Could you check a few things on this model? Use its own coordinates, in mm. A direction names the side the tool comes from. Coordinates: 2 decimals unless noted, no trailing zeros. Write each loop counter-clockwise with the first axis right and the second up, starting at its lowest first coordinate (ties: lowest second). Pieces come first, ordered by that corner, then holes. Notation, with made-up numbers: (1.25, 45) - (11.25, 45) arc R12 cw to (11.25, 54) - close; hole circle Ø9 at (78, 6). An arc over 180 degrees is marked (long way). Answer as a JSON object with one key per item and string values. Group by question number.
1) Will these pins go through, and if not, where does the flat tip stop? pin 1 Ø0.8 at (x, z) = (0, -2) entering from -Y; pin 2 Ø2 at (x, z) = (5, 2) entering from -Y; pin 3 Ø2 at (y, z) = (-5.5, -8) entering from +X.
2) We'd pull the mould along Z, two halves only. Please class faces 1 (the cylindrical face through (3.4, -4.1, 4.4)), 2 (the flat face through (0, -3, -10.5)), 3 (the flat face through (0, -7.5, -9)): released by +Z, released by -Z, zero draft, split by the parting line, or undercut.
3) If we section it at B-B (z = 4.5): Write out the boundary of the cut face in (x, y) (3 decimals), plus the area to 3 significant figures.
4) Please list where these lines run through material, in increasing order: line 1 along Z through (x, y) = (0, -5); line 2 along X through (y, z) = (-3.5, 6.25); line 3 along X through (y, z) = (-0.25, -4.75).
5) On a 3-axis mill with a long thin cutter (end or side, diameter ignored), from which of +Z, -Z, +X, -X, +Y, -Y can I reach the whole of each face in a straight line? I mean faces 4 (the flat face through (5, -0.8, 0)), 5 (the flat face through (0, -7.5, 9)), 6 (the flat face through (-5, -0.8, 0)), 7 (the cylindrical face through (1.5, -7.39, -4.44)). Say none if no direction works.
6) If we section it at D-D (y = -3.5): Write out the boundary of the cut face in (x, z).
7) If we section it at C-C (z = -9): Write out the boundary of the cut face in (x, y).
8) If we section it at A-A (x = 0): Write out the boundary of the cut face in (y, z) (3 decimals), plus the area to 3 significant figures.
```python
from build123d import *

# Parameters (mm, degrees)
EXTRUDE_1_DEPTH             = 10.5
FILLET_1_R                  = 0.3
FILLET_2_R                  = 2
HOLE_WIZARD_M82_D           = 6.8
HOLE_WIZARD_M82_CSINK_D     = 8.05
HOLE_WIZARD_M82_CSINK_ANGLE = 90


with BuildPart() as part:
    # Эскиз1 → Бобышка-Вытянуть1 (new body, symmetric)
    with BuildSketch(Plane.XY):
        with BuildLine():
            Line((-4, 0), (4, 0))
            Line((4, 0), (4, -0.8))
            Line((4, -0.8), (6.5, -0.8))
            Line((6.5, -0.8), (6.5, -1.6))
            ThreePointArc((6.5, -1.6), (4.386776199, -4.87777644), (1.5, -7.5))
            Line((1.5, -7.5), (-1.5, -7.5))
            ThreePointArc((-1.5, -7.5), (-4.386776199, -4.87777644), (-6.5, -1.6))
            Line((-6.5, -1.6), (-6.5, -0.8))
            Line((-6.5, -0.8), (-4, -0.8))
            Line((-4, -0.8), (-4, 0))
        make_face()
    extrude(amount=EXTRUDE_1_DEPTH, both=True)

    # Скругление1
    fillet_1_edges = [part.edges().sort_by_distance(p)[0] for p in [
        (6.5, -0.8, 0),
        (6.5, -1.6, 0),
        (-6.5, -1.6, 0),
        (-6.5, -0.8, 0),
        (-4, 0, 0),
        (4, 0, 0),
    ]]
    fillet(fillet_1_edges, radius=FILLET_1_R)

    # Скругление2
    fillet_2_edges = [part.edges().sort_by_distance(p)[0] for p in [
        (1.5, -7.5, 0),
        (-1.5, -7.5, 0),
    ]]
    fillet(fillet_2_edges, radius=FILLET_2_R)

    # Отверстие обработанное метчиком M82 (through all)
    with Locations(Plane(origin=(0, 0, 0), x_dir=(1, 0, 0), z_dir=(0, 1, 0))):
        with Locations((0, -4.5)):
            CounterSinkHole(HOLE_WIZARD_M82_D / 2, HOLE_WIZARD_M82_CSINK_D / 2, counter_sink_angle=HOLE_WIZARD_M82_CSINK_ANGLE)

    # Эскиз5 → Повернуть1 (revolve)
    with BuildSketch(Plane(origin=(0, 0, 0), x_dir=(0, 0, -1), z_dir=(1, 0, 0))):
        with BuildLine():
            Line((6.5, -4.3), (6.5, -8.3))
            ThreePointArc((6.5, -8.3), (4.5, -6.3), (6.5, -4.3))
        make_face()
    revolve(axis=Axis((0, -4.3, -6.5), (0, -1, 0)))


solid = part.part
```
Here are the results:
{
 "1": {"pin 1": "stops at y = -7.5", "pin 2": "stops at y = -5.32", "pin 3": "stops at x = 4.7"},
 "2": {"face 1": "undercut", "face 2": "released by -Z", "face 3": "zero draft"},
 "3": {"outline": "(-6.5, -1.532) arc R0.3 ccw to (-6.471, -1.662) arc R15 ccw to (-3.4, -5.934) - (-3.4, -0.625) - (-3.924, -0.101) arc R0.3 ccw to (-4, -0.3) - (-4, -0.8) - (-6.2, -0.8) arc R0.3 ccw to (-6.5, -1.1) - close; (3.4, -5.934) arc R15 ccw to (6.471, -1.662) arc R0.3 ccw to (6.5, -1.532) - (6.5, -1.1) arc R0.3 ccw to (6.2, -0.8) - (4, -0.8) - (4, -0.3) arc R0.3 ccw to (3.924, -0.101) - (3.4, -0.625) - close", "area": "20.6 mm²"},
 "4": {"line 1": "z = -10.5 to 1.1, 7.9 to 10.5", "line 2": "x = -5.42 to -2.92, 2.92 to 5.42", "line 3": "x = -4 to 4"},
 "5": {"face 4": "+Z, -Z, +X, +Y", "face 5": "+Z, +X, -X, -Y", "face 6": "+Z, -Z, -X, +Y", "face 7": "+X, -Y"},
 "6": {"outline": "(-5.42, -10.5) - (5.42, -10.5) - (5.42, 10.5) - (-5.42, 10.5) - close; hole circle Ø6.8 at (0, 4.5)"},
 "7": {"outline": "(-6.5, -1.53) arc R0.3 ccw to (-6.47, -1.66) arc R15 ccw to (-2.07, -7.09) arc R2 ccw to (-0.85, -7.5) - (0.85, -7.5) arc R2 ccw to (2.07, -7.09) arc R15 ccw to (6.47, -1.66) arc R0.3 ccw to (6.5, -1.53) - (6.5, -1.1) arc R0.3 ccw to (6.2, -0.8) - (4, -0.8) - (4, -0.3) arc R0.3 ccw to (3.7, 0) - (-3.7, 0) arc R0.3 ccw to (-4, -0.3) - (-4, -0.8) - (-6.2, -0.8) arc R0.3 ccw to (-6.5, -1.1) - close"},
 "8": {"outline": "(-7.5, -10.5) - (0, -10.5) - (0, 0.475) - (-0.625, 1.1) - (-7.5, 1.1) - (-7.5, -4.9) arc R2 ccw to (-7.5, -8.1) - close; (-7.5, 7.9) - (-0.625, 7.9) - (0, 8.525) - (0, 10.5) - (-7.5, 10.5) - close", "area": "108 mm²"}
}
